```python
from build123d import *

# Parameters (mm, degrees)
BOSS_EXTRUDE1_DEPTH = 127
SKETCH2_W           = 25.4
SKETCH2_H           = 6.35
SKETCH2_W_2         = 25.559422118
CUT_EXTRUDE1_DEPTH  = 6.35
CUT_EXTRUDE2_DEPTH  = 6.35
SKETCH4_R           = 2.0955
SKETCH4_R_2         = 1.828321723
CUT_EXTRUDE3_DEPTH  = 6.35


with BuildPart() as part:
    # Sketch1 → Boss-Extrude1 (new body)
    with BuildSketch(Plane.XY):
        Polygon((-127, 0), (0, -127), (4.490128061, -122.509871939), (-122.509871939, 4.490128061), align=None)
    extrude(amount=BOSS_EXTRUDE1_DEPTH)

    # Sketch2 → Cut-Extrude1 (cut)
    with BuildSketch(Plane(origin=(-63.5, -63.5, 0), x_dir=(0, 0, 1), z_dir=(-0.7071067811865509, -0.7071067811865441, 0))):
        with Locations((88.9, 86.627561211)):
            Rectangle(SKETCH2_W, SKETCH2_H)
        with Locations((38.020288941, 86.627561211)):
            Rectangle(SKETCH2_W_2, SKETCH2_H)
        with Locations((88.9, -86.627561211)):
            Rectangle(SKETCH2_W, SKETCH2_H)
        with Locations((38.020288941, -86.627561211)):
            Rectangle(SKETCH2_W_2, SKETCH2_H)
    extrude(amount=-CUT_EXTRUDE1_DEPTH, mode=Mode.SUBTRACT)

    # Sketch3 → Cut-Extrude2 (cut)
    with BuildSketch(Plane(origin=(-63.5, -63.5, 0), x_dir=(0, 0, 1), z_dir=(-0.7071067811865509, -0.7071067811865441, 0))):
        Polygon((91.0336, 83.452561211), (86.7664, 83.452561211), (86.7664, 74.689561211), (84.455, 74.689561211), (84.455, 71.514561211), (86.7664, 71.514561211), (86.7664, 68.212561211), (91.0336, 68.212561211), (91.0336, 71.514561211), (93.345, 71.514561211), (93.345, 74.689561211), (91.0336, 74.689561211), align=None)
        Polygon((40.153888941, 83.452561211), (35.886688941, 83.452561211), (35.886688941, 74.689561211), (33.575288941, 74.689561211), (33.575288941, 71.514561211), (35.886688941, 71.514561211), (35.886688941, 68.212561211), (40.153888941, 68.212561211), (40.153888941, 71.514561211), (42.465288941, 71.514561211), (42.465288941, 74.689561211), (40.153888941, 74.689561211), align=None)
        Polygon((86.7664, -83.452561211), (91.0336, -83.452561211), (91.0336, -74.689561211), (93.345, -74.689561211), (93.345, -71.514561211), (91.0336, -71.514561211), (91.0336, -68.212561211), (86.7664, -68.212561211), (86.7664, -71.514561211), (84.455, -71.514561211), (84.455, -74.689561211), (86.7664, -74.689561211), align=None)
        Polygon((35.886688941, -83.452561211), (40.153888941, -83.452561211), (40.153888941, -74.689561211), (42.465288941, -74.689561211), (42.465288941, -71.514561211), (40.153888941, -71.514561211), (40.153888941, -68.212561211), (35.886688941, -68.212561211), (35.886688941, -71.514561211), (33.575288941, -71.514561211), (33.575288941, -74.689561211), (35.886688941, -74.689561211), align=None)
    extrude(amount=-CUT_EXTRUDE2_DEPTH, mode=Mode.SUBTRACT)

    # Sketch4 → Cut-Extrude3 (cut)
    with BuildSketch(Plane(origin=(-59.009871939, -59.009871939, 0), x_dir=(0, 0, -1), z_dir=(0.707106781186551, 0.7071067811865441, 0))):
        with Locations(Location((-114.3, 86.627561211, 0), (0, 0, 90))):
            Circle(SKETCH4_R)
        with Locations(Location((-12.7, 86.627561211, 0), (0, 0, 90))):
            Circle(SKETCH4_R)
        with Locations(Location((-12.7, -86.627561211, 0), (0, 0, 90))):
            Circle(SKETCH4_R_2)
        with Locations(Location((-114.3, -86.627561211, 0), (0, 0, 90))):
            Circle(SKETCH4_R)
    extrude(amount=-CUT_EXTRUDE3_DEPTH, mode=Mode.SUBTRACT)


solid = part.part
```
Work out the finished part from the listing and answer in its coordinate system (mm). A direction names the side the tool comes from. Round coordinates to 2 decimals unless told otherwise and drop trailing zeros. Loops run counter-clockwise (first coordinate to the right, second up) from the corner with the lowest first, then second, coordinate; pieces in that order, holes last. Notation, with made-up numbers: M 5.25,79 L 26.25,79 A29 ccw 26.25,100 Z; hole C 33.25,-40 d3. An arc over 180 degrees is marked long. Use CSV: the item, a comma, the result in double quotes.
Q1. Each of these flat-tipped pins is pushed along its axis until it touches: pin 1 (8 mm diameter, centred on x = -98.5, z = 57.5, fed in from -Y); pin 2 (8 mm diameter, centred on y = -21, z = 51, fed in from +X); pin 3 (6 mm diameter, centred on x = -45.5, z = 25.5, fed in from -Y). Where does it stop, or does it pass through?
Determined:
pin 1,"y = -32.5"
pin 2,"x = -93.02"
pin 3,"y = -84.5"
Q2. Consider L1, parallel to Z at x = -7.5, y = -117; L2, parallel to Y at x = -84, z = 21; L3, parallel to Y at x = -82.5, z = 14. Determine where each line is inside the solid, lowest interval first.
Determined:
L1,"0 to 35.89, 40.15 to 86.77, 91.03 to 127"
L2,"-43 to -34.02"
L3,"-44.5 to -35.52"
Q3. Section A-A, the plane z = 63 is taken. Determine the outline of the cut face in (x, y), then the cut area to 3 significant figures.
Determined:
outline,"M -127,0 L 0,-127 L 4.49,-122.51 L -122.51,4.49 Z"
area,"1,140 mm2"
Q4. A tool of negligible diameter and unlimited length cuts with its end or side. For faces 1 (the flat face through (-10, -113, 33.575)), 2 (the flat face through (-5, -117, 40.154)), 3 (the flat face through (-111, -12, 40.154)), 4 (the flat face through (0, -123, 25.241)), from which of +Z, -Z, +X, -X, +Y, -Y can it reach the whole face along a straight path? Write none if from no direction.
Determined:
face 1,"none"
face 2,"+X, -X, +Y, -Y"
face 3,"-X, +Y"
face 4,"+X, -Y"
Q5. The mould has two halves that part along X. Classify faces 5 (the flat face through (-113, -10, 42.465)), 6 (the flat face through (-120.3, -2.28, 96.24)), 7 (the flat face through (-5, -117, 91.034)): pulls with the +X half, pulls with the -X half, needs draft (parallel to the pull), parting line crosses it, or undercut.
Determined:
face 5,"undercut"
face 6,"pulls with the -X half"
face 7,"needs draft"
Q6. Section B-B, the plane y = -74.5 is taken. Determine the outline of the cut face in (x, z).
Determined:
outline,"M -52.5,0 L -43.52,0 L -43.52,127 L -52.5,127 Z"
